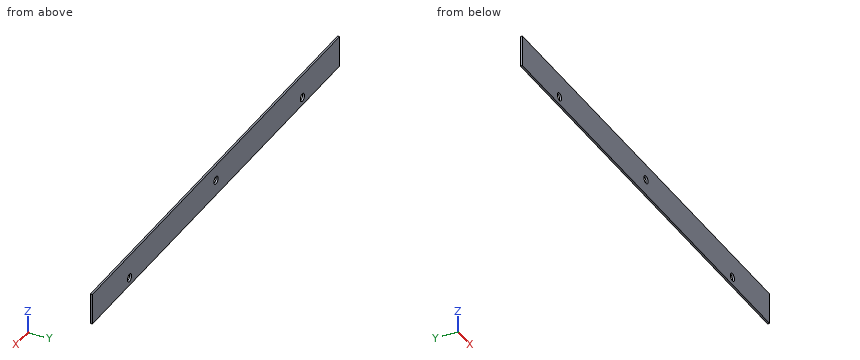
Autodesk Inventor part; units mm, degrees
ref_plane "YZ Plane" through (0, 0, 0) normal (1, 0, 0) x (0, 1, 0)
ref_plane "XZ Plane" through (0, 0, 0) normal (0, 1, 0) x (-1, 0, 0)
ref_plane "XY Plane" through (0, 0, 0) normal (0, 0, 1) x (1, 0, 0)
sketch "Sketch1" plane through (0, 0, 0) normal (0, 1, 0) x (-1, 0, 0)
  line L0 (0, 0) -> (762, 0)
  line L1 (762, 0) -> (762, 50.8)
  line L2 (762, 50.8) -> (0, 50.8)
  line L3 (0, 50.8) -> (0, 0)
  dimension "d0" = 762
  dimension "d1" = 50.8
extrude "Extrusion1" add sketch "Sketch1" along normal blind 3.175
sketch "Sketch2" plane through (0, 3.175, 0) normal (0, 1, 0) x (1, 0, 0)
  circle A0 centre (-381, -25.4) radius 6.35
  line L0 (0, 0) -> (-762, 0)
  line L1 (0, -50.8) -> (0, 0)
  circle A1 centre (-114.6026, -12.7) radius 6.35
  line L2 (-762, -50.8) -> (0, -50.8)
  circle A2 centre (-647.3974, -12.7) radius 6.35
  dimension "d4" = 12.7
  dimension "d5" = 25.4
  dimension "d6" = 381
  dimension "d9" = 12.7
  dimension "d10" = 38.1
  dimension "d11" = 266.7
  dimension "d12" = 12.7
  dimension "d13" = 38.1
  dimension "d14" = 266.7
extrude "Extrusion2" cut sketch "Sketch2" against normal blind 3.175
properties part number "side plate" material "Aluminum 6061"
The listing builds one solid part. Answer for the finished solid, in the listing's coordinates (mm). Round coordinates to 2 decimals unless told otherwise and drop trailing zeros. Loops run counter-clockwise (first coordinate to the right, second up) from the corner with the lowest first, then second, coordinate; pieces in that order, holes last.
Q1. Section B-B, the plane z = 25.4 is taken. Determine the outline of the cut face in (x, y) (3 decimals), then the cut area to 3 significant figures.
Q2. Given pin 1 Ø7.5 at (x, z) = (-114.6, 12.7) entering from -Y, flat-ended and moving along its own axis, determine where the tip first touches the part or whether it passes through.
Q3. Section A-A, the plane x = -381 is taken. Determine the outline of the cut face in (y, z) (3 decimals), then the cut area to 3 significant figures.
Q4. Find the intervals of material crossed by line 1 (X direction, y = 1.7, z = 12.7); line 2 (X direction, y = 1.75, z = 25.4); line 3 (X direction, y = 0.75, z = 10.5), in increasing order.
Completed:
1. outline: (-762, 0) - (-387.35, 0) - (-387.35, 3.175) - (-762, 3.175) - close; (-374.65, 0) - (0, 0) - (0, 3.175) - (-374.65, 3.175) - close
1. area: 2,380 mm2
2. pin 1: passes through
3. outline: (0, 0) - (3.175, 0) - (3.175, 19.05) - (0, 19.05) - close; (0, 31.75) - (3.175, 31.75) - (3.175, 50.8) - (0, 50.8) - close
3. area: 121 mm2
4. line 1: x = -762 to -653.75, -641.05 to -120.95, -108.25 to 0
4. line 2: x = -762 to -387.35, -374.65 to 0
4. line 3: x = -762 to -653.35, -641.44 to -120.56, -108.65 to 0
